Could you check a few things on this model? Use its own coordinates, in mm. Round coordinates to 2 decimals unless told otherwise and drop trailing zeros. Loops run counter-clockwise (first coordinate to the right, second up) from the corner with the lowest first, then second, coordinate; pieces in that order, holes last. Notation, with made-up numbers: M 81.25,21 L 86.25,21 A13 cw 86.25,40 Z; hole C 55,-22.75 d1. An arc over 180 degrees is marked long. One line per item, written item: value. Start each with the question number.
Q1. Thinking about a two-plate mould opening in X: for faces 1 (the face through (-83.154, 0.816, -1.972)), 2 (the face through (-91.002, 0.885, -1.972)), 3 (the face through (-87, -12, 0)), 4 (the face through (-87, 2, -2)), which applies, released by +X, released by -X, zero draft, split by the parting line, or undercut?
Q2. Please list where these lines run through material, in increasing order: line 1 along Y through (x, z) = (-87, -2.3); line 2 along Y through (x, z) = (-86, -2.75); line 3 along X through (y, z) = (-1.5, -3.8).
Q3. Imagine slicing it at C-C (x = -87.25). Please give me the cut outline in (y, z), then the cut area to 3 significant figures.
Q4. Imagine slicing it at A-A (z = -2). Please give me the cut outline in (x, y), then the cut area to 3 significant figures.
Q5. I'm going to push flat-ended pins straight in: pin 1 Ø1.5 at (x, z) = (-90, -2.5) entering from -Y; pin 2 Ø0.7 at (y, z) = (2.5, -2) entering from -X; pin 3 Ø2 at (x, z) = (-87.5, -1) entering from +Y. Where does each tip first touch, or does it pass through?
Q6. Imagine slicing it at B-B (x = -86). Please give me the cut outline in (y, z), then the cut area to 3 significant figures.
Autodesk Inventor part; units mm, degrees
ref_plane "YZ Plane" through (0, 0, 0) normal (1, 0, 0) x (0, 1, 0)
ref_plane "XZ Plane" through (0, 0, 0) normal (0, 1, 0) x (-1, 0, 0)
ref_plane "XY Plane" through (0, 0, 0) normal (0, 0, 1) x (1, 0, 0)
ref_plane "Work Plane1" through (0, 0, 0) normal (0, 0, 1) x (1, 0, 0)
sketch "Sketch1" plane through (0, 0, 0) normal (0, 0, 1) x (1, 0, 0)
  line L0 (227.5976, -2) -> (227.5976, -22)
  arc A0 (217.5976, -22) -> (227.5976, -22) centre (222.5976, -22) ccw
  line L1 (217.5976, -22) -> (217.5976, -2)
  arc A1 (227.5976, -2) -> (217.5976, -2) centre (222.5976, -2) ccw
  line L2 (78.8821, -22) -> (78.8821, -2)
  arc A2 (88.8821, -2) -> (78.8821, -2) centre (83.8821, -2) ccw
  line L3 (88.8821, -2) -> (88.8821, -22)
  arc A3 (78.8821, -22) -> (88.8821, -22) centre (83.8821, -22) ccw
  line L4 (-82.1032, -2) -> (-82.1032, -22)
  arc A4 (-92.1032, -22) -> (-82.1032, -22) centre (-87.1032, -22) ccw
  line L5 (-92.1032, -22) -> (-92.1032, -2)
  arc A5 (-82.1032, -2) -> (-92.1032, -2) centre (-87.1032, -2) ccw
  line L6 (374.3969, 34.0458) -> (374.3969, -61)
  line L7 (344.0734, 61) -> (374.3969, 34.0458)
  line L8 (-316.3526, 61) -> (344.0734, 61)
  line L9 (-354.2917, 27.0499) -> (-316.3526, 61)
  line L10 (-54.9688, -61) -> (-354.2917, 27.0499)
  line L11 (374.3969, -61) -> (-54.9688, -61)
  line L12 (-87.1032, -22) -> (-87.1032, -2) construction
  line L13 (-82.2532, -22) -> (-82.2532, -2)
  line L14 (-91.9532, -2) -> (-91.9532, -22)
  arc A6 (-91.9532, -22) -> (-82.2532, -22) centre (-87.1032, -22) ccw
  arc A7 (-82.2532, -2) -> (-91.9532, -2) centre (-87.1032, -2) ccw
  line L15 (-87.1032, 3) -> (-87.1032, 2)
  line L16 (-87.1032, 2) -> (-84.3605, 2)
  line L17 (-87.1032, 2) -> (-89.8459, 2)
  line L18 (-87.1032, 2) -> (-88.6032, 2)
  line L19 (-88.6032, 2) -> (-85.6032, 2)
  line L20 (-85.6032, 2) -> (-85.6032, 4.0639)
  line L21 (-88.6032, 2) -> (-88.6032, 3.4505)
  point P0 (0, 0)
  point P1 (-87.1032, -12)
  point P2 (-85.6032, 2.6122)
  point P3 (-88.6032, 2.6122)
  dimension "d0" = 9.7
  dimension "d1" = 1
  dimension "d2" = 1.5
  dimension "d3" = 3
extrude "Extrusion1" add sketch "Sketch1" against normal blind 4 contours A7 L16 L20 | A7 L13 A6 L14 L17 L16 | L21 L17 A7
properties part number "zaslepka_sruby_2"
Report:
1. face 1: released by +X
1. face 2: released by -X
1. face 3: zero draft
1. face 4: undercut
2. line 1: y = -26.85 to 2
2. line 2: y = -26.72 to 2
2. line 3: x = -91.93 to -82.28
3. outline: M -26.85,-4 L 2,-4 L 2,0 L -26.85,0 Z
3. area: 115 mm²
4. outline: M -91.95,-22 A4.85 ccw -82.25,-22 L -82.25,-2 A4.85 ccw -85.6,2.61 L -85.6,2 L -88.6,2 L -88.6,2.61 A4.85 ccw -91.95,-2 Z
4. area: 266 mm²
5. pin 1: stops at y = -26.35
5. pin 2: stops at x = -89.61
5. pin 3: stops at y = 2
6. outline: M -26.72,-4 L 2,-4 L 2,0 L -26.72,0 Z
6. area: 115 mm²
